```python
from build123d import *

# Parameters (mm, degrees)
BOSS_EXTRUDE1_DEPTH = 101.6
SKETCH2_R           = 3.175
CUT_EXTRUDE1_DEPTH  = 133.208158977


with BuildPart() as part:
    # Sketch1 → Boss-Extrude1 (new body)
    with BuildSketch(Plane(origin=(0, 0, 0), x_dir=(1, 0, 0), z_dir=(0, 1, 0))):
        with BuildLine():
            Line((55.518032206, 6.35), (68.58, 6.35))
            Line((68.58, 6.35), (68.58, 0))
            Line((68.58, 0), (49.53, 0))
            ThreePointArc((49.53, 0), (0, 49.53), (-49.53, 0))
            Line((-49.53, 0), (-68.58, 0))
            Line((-68.58, 0), (-68.58, 6.35))
            Line((-68.58, 6.35), (-55.518032206, 6.35))
            ThreePointArc((-55.518032206, 6.35), (0, 55.88), (55.518032206, 6.35))
        make_face()
    extrude(amount=BOSS_EXTRUDE1_DEPTH)

    # Sketch2 → Cut-Extrude1 (cut, through all)
    with BuildSketch(Plane(origin=(0, 0, -6.35), x_dir=(-1, 0, 0), z_dir=(0, 0, -1))):
        with Locations((62.049016103, 88.9)):
            Circle(SKETCH2_R)
        with Locations((62.049016103, 63.5)):
            Circle(SKETCH2_R)
        with Locations((62.049016103, 38.1)):
            Circle(SKETCH2_R)
        with Locations((62.049016103, 12.7)):
            Circle(SKETCH2_R)
        with Locations(Location((-62.049016103, 12.7, 0), (0, 0, 180))):
            Circle(SKETCH2_R)
        with Locations(Location((-62.049016103, 38.1, 0), (0, 0, 180))):
            Circle(SKETCH2_R)
        with Locations(Location((-62.049016103, 63.5, 0), (0, 0, 180))):
            Circle(SKETCH2_R)
        with Locations(Location((-62.049016103, 88.9, 0), (0, 0, 180))):
            Circle(SKETCH2_R)
    extrude(amount=-CUT_EXTRUDE1_DEPTH, mode=Mode.SUBTRACT)


solid = part.part
```
Check sheet for the modelled part. Datum: model origin and axes. Units: mm. A direction names the side the tool comes from. Coordinates: 2 decimals unless noted, no trailing zeros. Loops run counter-clockwise (first coordinate to the right, second up) from the corner with the lowest first, then second, coordinate; pieces in that order, holes last. Notation, with made-up numbers: M 22,-24 L 68,-24 A34 ccw 68,14 Z; hole C 70.5,64.25 d2. An arc over 180 degrees is marked long. Answer as a JSON object with one key per item and string values.
1. Sectioned sample at D-D on z = -39. Record the cut outline in (x, y).
Outcome:
{"outline": "M -40.02,0 L -30.53,0 L -30.53,101.6 L -40.02,101.6 Z; M 30.53,0 L 40.02,0 L 40.02,101.6 L 30.53,101.6 Z"}
2. Sectioned sample at C-C on x = 0. Record the cut outline in (y, z).
Outcome:
{"outline": "M 0,-55.88 L 101.6,-55.88 L 101.6,-49.53 L 0,-49.53 Z"}
3. Depth check by flat-ended pin: P1, Ø4, axis at x = -37.5, y = 81, coming from the -Z side; P2, Ø10, axis at y = 11, z = -48.5, coming from the +X side; P3, Ø6, axis at x = -19, y = 18.5, coming from the -Z side. Enter the tip coordinate at first touch or a pass-through.
Outcome:
{"P1": "z = -43.15", "P2": "x = 35.08", "P3": "z = -53.54"}
4. Scan lines: L1, parallel to X at y = 58, z = -39.5; L2, parallel to X at y = 70.5, z = -19; L3, parallel to Z at x = -1, y = 45. Record each from-to range of solid material in increasing order. Write a range as from..to.
Outcome:
{"L1": "-39.53..-29.88, 29.88..39.53", "L2": "-52.55..-45.74, 45.74..52.55", "L3": "-55.87..-49.52"}
5. Release check for a two-part mould opening along Y. For faces 1 (the flat face through (59, 50, 0)), 2 (the cylindrical face through (65.08, 62.55, -3.22)), 3 (the flat face through (0, 0, -51)) record: pulls with the +Y half, pulls with the -Y half, needs draft (parallel to the pull), parting line crosses it, or undercut.
Outcome:
{"face 1": "needs draft", "face 2": "undercut", "face 3": "pulls with the -Y half"}
6. Sectioned sample at B-B on z = -14. Record the cut outline in (x, y), and give its area (3 significant figures).
Outcome:
{"outline": "M -54.1,0 L -47.51,0 L -47.51,101.6 L -54.1,101.6 Z; M 47.51,0 L 54.1,0 L 54.1,101.6 L 47.51,101.6 Z", "area": "1,340 mm²"}
7. Access from +Z, -Z, +X, -X, +Y, -Y to the whole of each face (thin tool, end or side, straight path). Record for faces 4 (the flat face through (-59, 50, 0)), 5 (the flat face through (62, 50, -6.35)), 6 (the flat face through (-62, 50, -6.35)).
Outcome:
{"face 4": "+Z, +X, -X, +Y, -Y", "face 5": "-Z, +X, +Y, -Y", "face 6": "-Z, -X, +Y, -Y"}
8. Sectioned sample at A-A on y = 38.1. Record the cut outline in (x, z), and give its area (3 significant figures).
Outcome:
{"outline": "M -68.58,-6.35 L -65.22,-6.35 L -65.22,0 L -68.58,0 Z; M -58.87,-6.35 L -55.52,-6.35 A55.88 ccw 55.52,-6.35 L 58.87,-6.35 L 58.87,0 L 49.53,0 A49.53 cw -49.53,0 L -58.87,0 Z; M 65.22,-6.35 L 68.58,-6.35 L 68.58,0 L 65.22,0 Z", "area": "1,130 mm²"}
